from build123d import *

# Parameters (mm, degrees)
F1_DEPTH = 6.985
F2_R     = 0.762
F3_R     = 0.762


with BuildPart() as f1:
    # F0 (on Top) → F1 (new body)
    with BuildSketch(Plane.XY):
        with BuildLine():
            ThreePointArc((0, 11.0109), (7.785882, 7.785882), (11.0109, 0))
            ThreePointArc((11.0109, 0), (7.785882, -7.785882), (0, -11.0109))
            Line((0, -11.0109), (0, -13.97))
            ThreePointArc((0, -13.97), (11.674333, -18.805667), (16.51, -30.48))
            Line((16.51, -30.48), (16.51, 30.48))
            ThreePointArc((16.51, 30.48), (11.674333, 18.805667), (0, 13.97))
            Line((0, 13.97), (0, 11.0109))
        make_face()
        with BuildLine():
            ThreePointArc((0, -11.0109), (-11.0109, 0), (0, 11.0109))
            Line((0, 11.0109), (0, 13.97))
            ThreePointArc((0, 13.97), (-11.674333, 18.805667), (-16.51, 30.48))
            Line((-16.51, 30.48), (-16.51, -30.48))
            ThreePointArc((-16.51, -30.48), (-11.674333, -18.805667), (0, -13.97))
            Line((0, -13.97), (0, -11.0109))
        make_face()
        with BuildLine():
            ThreePointArc((11.0109, 30.48), (-7.785882, 38.265882), (0, 19.4691))
            ThreePointArc((0, 19.4691), (7.785882, 22.694118), (11.0109, 30.48))
        make_face()
        with BuildLine():
            ThreePointArc((-16.51, 30.48), (-11.674333, 18.805667), (0, 13.97))
            ThreePointArc((0, 13.97), (11.674333, 18.805667), (16.51, 30.48))
            ThreePointArc((16.51, 30.48), (0, 46.99), (-16.51, 30.48))
        make_face()
        with BuildLine():
            ThreePointArc((11.0109, 30.48), (7.785882, 22.694118), (0, 19.4691))
            ThreePointArc((0, 19.4691), (-7.785882, 38.265882), (11.0109, 30.48))
        make_face(mode=Mode.SUBTRACT)
        with BuildLine():
            ThreePointArc((11.0109, -30.48), (7.785882, -22.694118), (0, -19.4691))
            ThreePointArc((0, -19.4691), (-7.785882, -38.265882), (11.0109, -30.48))
        make_face()
        with BuildLine():
            ThreePointArc((16.51, -30.48), (11.674333, -18.805667), (0, -13.97))
            ThreePointArc((0, -13.97), (-11.674333, -18.805667), (-16.51, -30.48))
            ThreePointArc((-16.51, -30.48), (0, -46.99), (16.51, -30.48))
        make_face()
        with BuildLine():
            ThreePointArc((11.0109, -30.48), (-7.785882, -38.265882), (0, -19.4691))
            ThreePointArc((0, -19.4691), (7.785882, -22.694118), (11.0109, -30.48))
        make_face(mode=Mode.SUBTRACT)
    extrude(amount=F1_DEPTH)

    # F2
    f2_edges = [f1.edges().sort_by_distance(p)[0] for p in [
        (16.51, 0, 6.985),
    ]]
    fillet(f2_edges, radius=F2_R)

    # F3
    f3_edges = [f1.edges().sort_by_distance(p)[0] for p in [
        (0, -46.99, 0),
        (16.51, 0, 0),
        (-16.51, 30.48, 3.1115),
        (-16.51, 0, 0),
    ]]
    fillet(f3_edges, radius=F3_R)


solid = f1.part
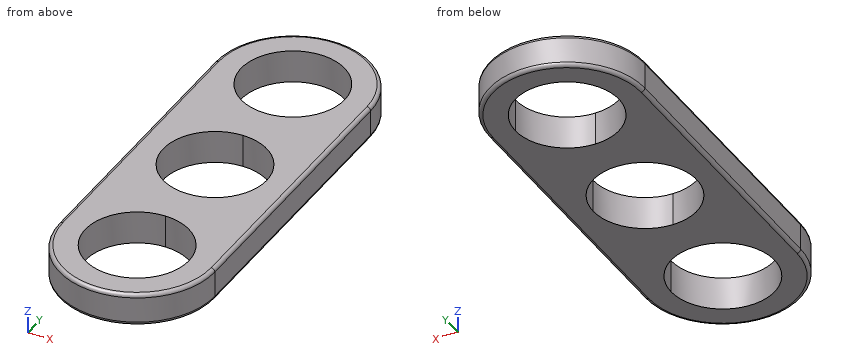
Build history of the part. All positions in model axes, mm. Round coordinates to 2 decimals unless told otherwise and drop trailing zeros. Write each loop counter-clockwise with the first axis right and the second up, starting at its lowest first coordinate (ties: lowest second). Pieces come first, ordered by that corner, then holes. Notation, with made-up numbers: M -12,67.25 L 22,67.25 A12 ccw 22,73.25 Z; hole C 89.25,71 d2. An arc over 180 degrees is marked long. Answer as a JSON object with one key per item and string values. Group by question number.
(1) Cut at B-B (y = 25). Give the cut face in (x, z) (3 decimals), and give its area (3 significant figures).
(2) Flat gauge pins, fed straight in: pin 1 (4 mm diameter, centred on y = 31, z = 5, fed in from -X); pin 2 (1.5 mm diameter, centred on x = -11, z = 5.5, fed in from +Y); pin 3 (3 mm diameter, centred on x = -10, z = 5.5, fed in from +Y). Where does each tip first touch, or does it go through?
(3) Cut at A-A (z = 1.75). Give the cut face in (x, y).
(4) Drill centre lines: L1, parallel to X at y = -30.48, z = 2.25; L2, parallel to Y at x = 7, z = 6; L3, parallel to Y at x = 6, z = 6.5. Where is each one in solid material? Low to high.
(5) Cut at D-D (x = 2). Give the number of separate pieces and of enclosed holes in the cut face, and give its area (3 significant figures).
(6) Cut at C-C (y = -9). Give the cut face in (x, z) (1 decimal), and give its area (3 significant figures).
Responses:
{
 "1": {"outline": "M -16.51,0.762 A0.762 ccw -15.748,0 L -9.55,0 L -9.55,6.985 L -15.748,6.985 A0.762 ccw -16.51,6.223 Z; M 9.55,0 L 15.748,0 A0.762 ccw 16.51,0.762 L 16.51,6.223 A0.762 ccw 15.748,6.985 L 9.55,6.985 Z", "area": "96.7 mm2"},
 "2": {"pin 1": "stops at x = -16.51", "pin 2": "stops at y = 43.42", "pin 3": "stops at y = 44.63"},
 "3": {"outline": "M -16.51,-30.48 A16.51 ccw 16.51,-30.48 L 16.51,30.48 A16.51 ccw -16.51,30.48 Z; hole C 0,-30.48 d22.02; hole C 0,0 d22.02; hole C 0,30.48 d22.02"},
 "4": {"L1": "x = -16.51 to -11.01, 11.01 to 16.51", "L2": "y = -45.43 to -38.98, -21.98 to -8.5, 8.5 to 21.98, 38.98 to 45.43", "L3": "y = -45.81 to -39.71, -21.25 to -9.23, 9.23 to 21.25, 39.71 to 45.81"},
 "5": {"separate pieces": "4", "enclosed holes": "0", "area": "200 mm2"},
 "6": {"outline": "M -16.5,0.8 A0.8 ccw -15.7,0 L -6.3,0 L -6.3,7 L -15.7,7 A0.8 ccw -16.5,6.2 Z; M 6.3,0 L 15.7,0 A0.8 ccw 16.5,0.8 L 16.5,6.2 A0.8 ccw 15.7,7 L 6.3,7 Z", "area": "142 mm2"}
}
